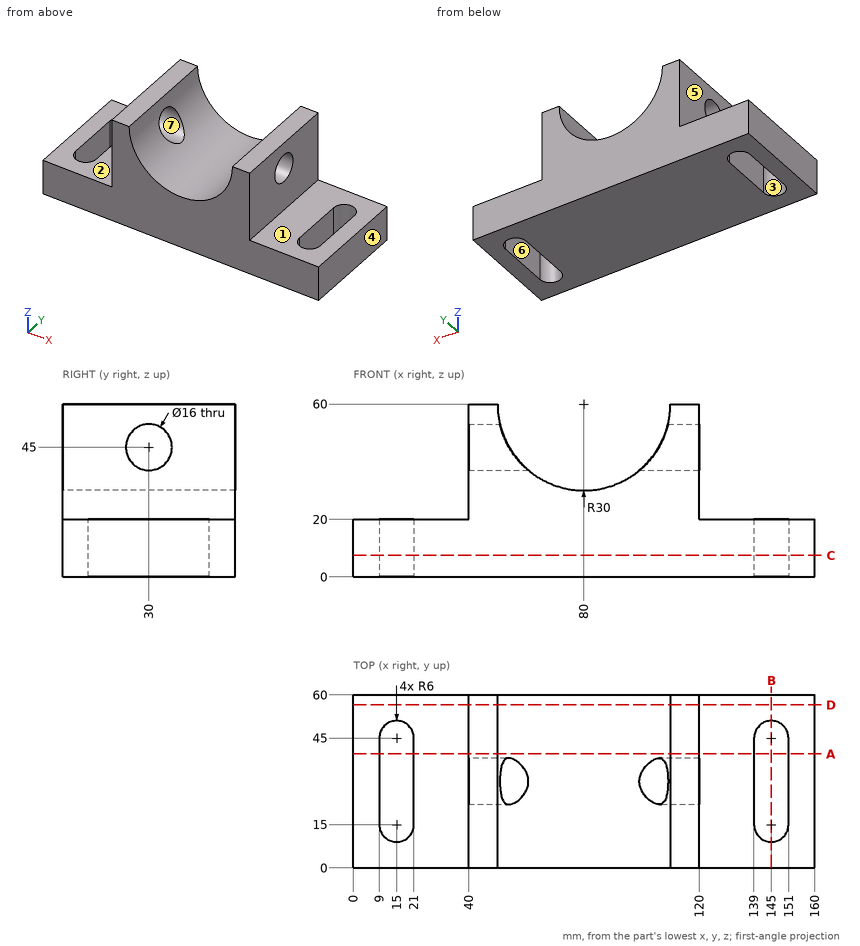
Check sheet for the drawn part. Datum: minimum x, y, z corner. Units: mm. A direction names the side the tool comes from. Round coordinates to 2 decimals unless told otherwise and drop trailing zeros. Write each loop counter-clockwise with the first axis right and the second up, starting at its lowest first coordinate (ties: lowest second). Pieces come first, ordered by that corner, then holes. Notation, with made-up numbers: (27, -0.5) -> (55, -0.5) arc R19 cw to (55, 35.5) -> close; hole circle Ø4 at (78.5, 61.25). An arc over 180 degrees is marked (long way). Put each result on its own line as item: value.
(1) Sectioned sample at A-A (y = 39.5). Enter the section's corners in (x, z), plus the area to 3 significant figures.
Values found:
outline: (0, 0) -> (9, 0) -> (9, 20) -> (0, 20) -> close; (21, 0) -> (139, 0) -> (139, 20) -> (120, 20) -> (120, 60) -> (110, 60) arc R30 cw to (50, 60) -> (40, 60) -> (40, 20) -> (21, 20) -> close; (151, 0) -> (160, 0) -> (160, 20) -> (151, 20) -> close
area: 4,510 mm^2
(2) Sectioned sample at D-D (y = 56.5). Enter the section's corners in (x, z).
Values found:
outline: (0, 0) -> (160, 0) -> (160, 20) -> (120, 20) -> (120, 60) -> (110, 60) arc R30 cw to (50, 60) -> (40, 60) -> (40, 20) -> (0, 20) -> close
(3) Go/stop test with flat-tipped pins: pin 1 Ø3 at (y, z) = (19, 25.5) entering from -X; pin 2 Ø20 at (x, y) = (21, 29) entering from +Z; pin 3 Ø20 at (y, z) = (23.5, 46) entering from +X. Record where each tip stops, or that it passes through.
Values found:
pin 1: stops at x = 40
pin 2: stops at z = 20
pin 3: stops at x = 120
(4) Sectioned sample at B-B (x = 145). Enter the section's corners in (y, z).
Values found:
outline: (0, 0) -> (9, 0) -> (9, 20) -> (0, 20) -> close; (51, 0) -> (60, 0) -> (60, 20) -> (51, 20) -> close
(5) Material ranges on line 1 (X direction, y = 21.5, z = 2.5); line 2 (Y direction, x = 47, z = 45); line 3 (Z direction, x = 113, y = 30), recorded low to high.
Values found:
line 1: x = 0 to 9, 21 to 139, 151 to 160
line 2: y = 0 to 22, 38 to 60
line 3: z = 0 to 37, 53 to 60
(6) Mould release check, pull along X, two halves, no side actions. Record for the marked faces 4, 5, 6 and 7: released by +X, released by -X, zero draft, split by the parting line, or undercut.
Values found:
face 4: released by +X
face 5: released by -X
face 6: undercut
face 7: zero draft
(7) Tool access check on the marked faces 1, 2 and 3. Record the directions out of +Z, -Z, +X, -X, +Y, -Y that give a thin tool (end or side, any length) a straight path to the whole face; none if there is none.
Values found:
face 1: +Z, +X, +Y, -Y
face 2: +Z, -X, +Y, -Y
face 3: +Z, -Z
(8) Sectioned sample at C-C (z = 7.5). Enter the section's corners in (x, y).
Values found:
outline: (0, 0) -> (160, 0) -> (160, 60) -> (0, 60) -> close; hole (9, 15) arc R6 ccw to (21, 15) -> (21, 45) arc R6 ccw to (9, 45) -> close; hole (139, 15) arc R6 ccw to (151, 15) -> (151, 45) arc R6 ccw to (139, 45) -> close
